Autodesk Inventor part; units mm, degrees
ref_plane "YZ Plane" through (0, 0, 0) normal (1, 0, 0) x (0, 1, 0)
ref_plane "XZ Plane" through (0, 0, 0) normal (0, 1, 0) x (-1, 0, 0)
ref_plane "XY Plane" through (0, 0, 0) normal (0, 0, 1) x (1, 0, 0)
sketch "Sketch1" plane through (0, 0, 0) normal (0, 0, 1) x (1, 0, 0)
  line L0 (0, 0) -> (330, 0)
  line L1 (330, 0) -> (330, 497)
  line L2 (330, 497) -> (0, 497)
  line L3 (0, 497) -> (0, 0)
  dimension "d0" = 330
  dimension "d1" = 497
extrude "Extrusion1" add sketch "Sketch1" along normal blind 10
sketch "Sketch2" plane through (0, 0, 10) normal (0, 0, 1) x (1, 0, 0)
  line L0 (0, 0) -> (330, 0)
  line L1 (330, 0) -> (330, 497)
  line L2 (330, 497) -> (0, 497)
  line L3 (0, 497) -> (0, 0)
  line L4 (10, 487) -> (320, 487)
  line L5 (320, 487) -> (320, 10)
  line L6 (320, 10) -> (10, 10)
  line L7 (10, 10) -> (10, 487)
  dimension "d4" = 330
  dimension "d5" = 497
  dimension "d6" = 10
extrude "Extrusion2" add sketch "Sketch2" along normal blind 177
properties part number "box_under"
Verification items for the finished model (mm, model axes). A direction names the side the tool comes from. Give positions to 0.01 mm unless a question says otherwise; leave off trailing zeros. Loops run counter-clockwise (first coordinate to the right, second up) from the corner with the lowest first, then second, coordinate; pieces in that order, holes last. Notation, with made-up numbers: (49.25, 77.5) - (78.25, 77.5) arc R21 cw to (78.25, 106.5) - close; hole circle Ø7 at (65, -11.5). An arc over 180 degrees is marked (long way). Write item = value, one per line. Start each with the question number.
Q1. Thickness scan on line 1 (X direction, y = 454.5, z = 127); line 2 (Y direction, x = 239.5, z = 30); line 3 (Z direction, x = 185.5, y = 29). Record the ranges inside material, lowest first.
Q2. Tool access check on faces 4 (the face through (330, 245, 92)), 5 (the face through (167, 10, 97)). Record the directions out of +Z, -Z, +X, -X, +Y, -Y that give a thin tool (end or side, any length) a straight path to the whole face; none if there is none.
Q3. Cross-section at C-C, the plane x = 244.5. Enter the section's corners in (y, z).
Q4. Cross-section at A-A, the plane z = 47. Enter the section's corners in (x, y), and give its area (3 significant figures).
Q5. Mould release check, pull along X, two halves, no side actions. Record for faces 1 (the face through (163, 252, 0)), 2 (the face through (0, 252, 92)), 3 (the face through (10, 245, 97)): released by +X, released by -X, zero draft, split by the parting line, or undercut.
Q6. Depth check by flat-ended pin: P1, Ø2, axis at x = 154.5, y = 60.5, coming from the +Z side. Enter the tip coordinate at first touch or a pass-through.
Q7. Cross-section at B-B, the plane y = 105.5. Enter the section's corners in (x, z).
Answer key:
q1.line_1 = 0 to 10, 320 to 330
q1.line_2 = 0 to 10, 487 to 497
q1.line_3 = 0 to 10
q2.face_4 = +Z, -Z, +X, +Y, -Y
q2.face_5 = +Z
q3.outline = (0, 0) - (497, 0) - (497, 187) - (487, 187) - (487, 10) - (10, 10) - (10, 187) - (0, 187) - close
q4.outline = (0, 0) - (330, 0) - (330, 497) - (0, 497) - close; hole (10, 10) - (320, 10) - (320, 487) - (10, 487) - close
q4.area = 16,100 mm^2
q5.face_1 = zero draft
q5.face_2 = released by -X
q5.face_3 = undercut
q6.P1 = 10
q7.outline = (0, 0) - (330, 0) - (330, 187) - (320, 187) - (320, 10) - (10, 10) - (10, 187) - (0, 187) - close
